The model under review builds one solid part; all positions refer to its coordinate system, in mm. Face numbers are marked on the shaded views. A direction names the side the tool comes from. Coordinates: 2 decimals unless noted, no trailing zeros. Loops run counter-clockwise (first coordinate to the right, second up) from the corner with the lowest first, then second, coordinate; pieces in that order, holes last. Notation, with made-up numbers: M 73.25,16 L 131.25,16 A20 cw 131.25,20 Z; hole C 31.25,-8 d5. An arc over 180 degrees is marked long. Return JSON: item names as keys, results as strings.
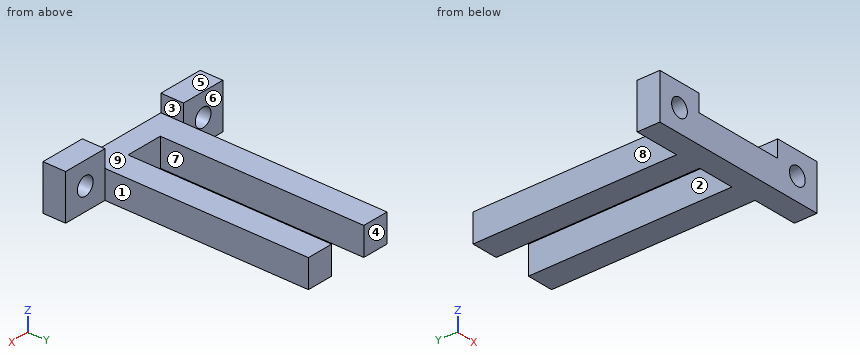
```python
from build123d import *

# Parameters (mm, degrees)
SKETCH_2_W          = 5.9
SKETCH_2_H          = 6.2
EXTRUDE_1_DEPTH     = 50
EXTRUDE_1_2_DEPTH   = 50
SKETCH_3_W          = 40
SKETCH_3_H          = 6.2
EXTRUDE_2_DEPTH     = 5
SKETCH_4_W          = 10
SKETCH_4_H          = 5
EXTRUDE_3_DEPTH     = 3.8
CUT_EXTRUDE_4_REACH = 56.437
SKETCH_5_R          = 2


with BuildPart() as part:
    # Sketch 2 → Extrude 1 (new body)
    with BuildSketch(Plane(origin=(0, 0, 0), x_dir=(1, 0, 0), z_dir=(0, 1, 0))):
        with Locations((2.95, 3.1)):
            Rectangle(SKETCH_2_W, SKETCH_2_H)
    extrude(amount=EXTRUDE_1_DEPTH)



with BuildPart() as body_2:
    # Sketch 2 → Extrude 1 2 (new body)
    with BuildSketch(Plane(origin=(0, 0, 0), x_dir=(1, 0, 0), z_dir=(0, 1, 0))):
        with Locations((17.05, 3.1)):
            Rectangle(SKETCH_2_W, SKETCH_2_H)
    extrude(amount=EXTRUDE_1_2_DEPTH)


with BuildPart() as part_1:
    add(part.part)

    add(body_2.part)  # Extrude 2 merges body 2
    # Sketch 3 → Extrude 2 (add)
    with BuildSketch(Plane(origin=(0, 0, 0), x_dir=(1, 0, 0), z_dir=(0, 1, 0))):
        with Locations((10, 3.1)):
            Rectangle(SKETCH_3_W, SKETCH_3_H)
    extrude(amount=EXTRUDE_2_DEPTH)

    # Sketch 4 → Extrude 3 (add)
    with BuildSketch(Plane.XY):
        with Locations((-5, 2.5)):
            Rectangle(SKETCH_4_W, SKETCH_4_H)
        with Locations((25, 2.5)):
            Rectangle(SKETCH_4_W, SKETCH_4_H)
    extrude(amount=EXTRUDE_3_DEPTH)

    # Sketch 5 → Cut-Extrude 4 (cut, up to next)
    with BuildSketch(Plane(origin=(0, 5, 0), x_dir=(1, 0, 0), z_dir=(0, 1, 0)), mode=Mode.PRIVATE) as cut_extrude_4_sk1:
        with Locations(Location((25, 1.2, 0), (0, 0, 270))):
            Circle(SKETCH_5_R)
    cut_extrude_4_tool1 = extrude(cut_extrude_4_sk1.sketch, amount=-CUT_EXTRUDE_4_REACH, mode=Mode.PRIVATE) & part_1.part
    # Sketch 5 → Cut-Extrude 4 (cut, up to next)
    with BuildSketch(Plane(origin=(0, 5, 0), x_dir=(1, 0, 0), z_dir=(0, 1, 0)), mode=Mode.PRIVATE) as cut_extrude_4_sk2:
        with Locations(Location((-5, 1.2, 0), (0, 0, 270))):
            Circle(SKETCH_5_R)
    cut_extrude_4_tool2 = extrude(cut_extrude_4_sk2.sketch, amount=-CUT_EXTRUDE_4_REACH, mode=Mode.PRIVATE) & part_1.part
    add(cut_extrude_4_tool1.solids().sort_by_distance((25, 5, -1.2))[0], mode=Mode.SUBTRACT)
    add(cut_extrude_4_tool2.solids().sort_by_distance((-5, 5, -1.2))[0], mode=Mode.SUBTRACT)


solid = part_1.part
```
1. Add section A-A on z = 1.5. Give the boundary of the cut face in (x, y), plus the area to 3 significant figures.
Check values:
{"outline": "M -10,0 L 0,0 L 0,5 L -10,5 Z; M 20,0 L 30,0 L 30,5 L 20,5 Z", "area": "100 mm²"}
2. Insertion check: pin 1 Ø5 at (y, z) = (37, -1.5) entering from -X; pin 2 Ø8 at (x, y) = (0.5, 33) entering from +Z; pin 3 Ø1 at (y, z) = (34, 0) entering from +X. Each pin has a flat end and moves straight along its axis. Give the tip position at first contact, or say it passes through.
Check values:
{"pin 1": "x = 0", "pin 2": "z = 0", "pin 3": "x = 20"}
3. Add section D-D on y = 3.5. Give the boundary of the cut face in (x, z), plus the area to 3 significant figures.
Check values:
{"outline": "M -10,-6.2 L 30,-6.2 L 30,3.8 L 20,3.8 L 20,0 L 0,0 L 0,3.8 L -10,3.8 Z; hole C -5,-1.2 d4; hole C 25,-1.2 d4", "area": "299 mm²"}
4. To check wall thickness, follow line 1 (X direction, y = 1.8, z = -1.2); line 2 (X direction, y = 22.5, z = -1.25); line 3 (Y direction, x = 25, z = -5). State the ranges of each line that lie inside material, in increasing order.
Check values:
{"line 1": "-10 to -7, -3 to 23, 27 to 30", "line 2": "0 to 5.9, 14.1 to 20", "line 3": "0 to 5"}
5. Add section C-C on z = -1.2. Give the boundary of the cut face in (x, y), plus the area to 3 significant figures.
Check values:
{"outline": "M -10,0 L -7,0 L -7,5 L -10,5 Z; M -3,0 L 23,0 L 23,5 L 20,5 L 20,50 L 14.1,50 L 14.1,5 L 5.9,5 L 5.9,50 L 0,50 L 0,5 L -3,5 Z; M 27,0 L 30,0 L 30,5 L 27,5 Z", "area": "691 mm²"}
6. Machinability: for the marked faces 1, 2, 3, 4 and 5, which of the approach directions +Z, -Z, +X, -X, +Y, -Y give a long, thin tool a straight path to every point of the face, cutting with its end or side? Answer none if there is none.
Check values:
{"face 1": "+Z, -Z, +X, +Y", "face 2": "+Z, -Z, +Y", "face 3": "+Z, +Y, -Y", "face 4": "+Z, -Z, +X, -X, +Y", "face 5": "+Z, +X, -X, +Y, -Y"}
7. Add section B-B on x = -5. Give the boundary of the cut face in (y, z).
Check values:
{"outline": "M 0,-6.2 L 5,-6.2 L 5,-3.2 L 0,-3.2 Z; M 0,0.8 L 5,0.8 L 5,3.8 L 0,3.8 Z"}
8. The part is to be moulded in two halves that separate along X. For the marked faces 6, 7, 8 and 9, say which applies: released by +X, released by -X, zero draft, split by the parting line, or undercut.
Check values:
{"face 6": "zero draft", "face 7": "undercut", "face 8": "released by -X", "face 9": "undercut"}
